Could you check a few things on this model? Use its own coordinates, in mm. A direction names the side the tool comes from. Coordinates: 2 decimals unless noted, no trailing zeros.
from build123d import *

# Parameters (mm, degrees)
F1_DEPTH = 25
F2_D     = 28
F2_DEPTH = 17
F2_TIP   = 8.4120486664
F3_D     = 28
F3_DEPTH = 17
F3_TIP   = 8.4120486664
F4_R     = 10
F5_DEPTH = 25


with BuildPart() as f1:
    # F0 (on Front) → F1 (new body)
    with BuildSketch(Plane.XZ):
        with BuildLine():
            Line((-279.2028378171, 167.9137703829), (54.3474347586, 546.1242293713))
            ThreePointArc((54.3474347586, 546.1242293713), (45.905243427, 563.8289204578), (52.8386613021, 582.1770647105))
            Line((52.8386613021, 582.1770647105), (-362.0687545083, 149.4799000496))
            ThreePointArc((-362.0687545083, 149.4799000496), (-347.0310263397, 160.2264674692), (-329.1166074138, 164.7757063423))
            Line((-329.1166074138, 164.7757063423), (-279.2028378171, 167.9137703829))
        make_face()
        with BuildLine():
            ThreePointArc((70.8833804527, 539.8742293713), (62.0445456879, 541.488870704), (54.3474347586, 546.1242293713))
            Line((54.3474347586, 546.1242293713), (-279.2028378171, 167.9137703829))
            Line((-279.2028378171, 167.9137703829), (-215.3865282422, 171.9258830303))
            Line((-215.3865282422, 171.9258830303), (-35.7808883073, 393.5494389695))
            Line((-35.7808883073, 393.5494389695), (70.8833804527, 525.16732437))
            Line((70.8833804527, 525.16732437), (70.8833804527, 539.8742293713))
        make_face()
        with BuildLine():
            Line((-215.3865282422, 171.9258830303), (-279.2028378171, 167.9137703829))
            Line((-279.2028378171, 167.9137703829), (-292.9074248186, 152.3742293713))
            ThreePointArc((-292.9074248186, 152.3742293713), (-281.7851423828, 138.2595880387), (-276.3714791245, 121.1242293713))
            Line((-276.3714791245, 121.1242293713), (-254.3034374995, 123.904541279))
            Line((-254.3034374995, 123.904541279), (-215.3865282422, 171.9258830303))
        make_face()
        with BuildLine():
            Line((-35.7808883073, 393.5494389695), (-215.3865282422, 171.9258830303))
            Line((-215.3865282422, 171.9258830303), (69.3147348493, 189.8249678568))
            ThreePointArc((69.3147348493, 189.8249678568), (-49.7750455866, 257.3601064033), (-35.7808883073, 393.5494389695))
        make_face()
        with BuildLine():
            Line((54.3474347586, 546.1242293713), (61.788610321, 554.5617293713))
            ThreePointArc((61.788610321, 554.5617293713), (65.226110321, 577.4064995031), (84.6333804527, 564.8742293713))
            ThreePointArc((84.6333804527, 564.8742293713), (80.6060986941, 555.15151113), (70.8833804527, 551.1242293713))
            Line((70.8833804527, 551.1242293713), (70.8833804527, 539.8742293713))
            ThreePointArc((70.8833804527, 539.8742293713), (81.64190304, 542.3075683037), (90.3060950779, 549.1338940322))
            ThreePointArc((90.3060950779, 549.1338940322), (94.4478437994, 556.5246145787), (95.8833804527, 564.8742293713))
            ThreePointArc((95.8833804527, 564.8742293713), (80.2075968068, 588.0703279524), (52.8386613021, 582.1770647105))
            ThreePointArc((52.8386613021, 582.1770647105), (45.905243427, 563.8289204578), (54.3474347586, 546.1242293713))
        make_face()
        with BuildLine():
            ThreePointArc((70.8833804527, 551.1242293713), (66.0220213321, 552.0122821043), (61.788610321, 554.5617293713))
            Line((61.788610321, 554.5617293713), (54.3474347586, 546.1242293713))
            ThreePointArc((54.3474347586, 546.1242293713), (62.0445456879, 541.488870704), (70.8833804527, 539.8742293713))
            Line((70.8833804527, 539.8742293713), (70.8833804527, 551.1242293713))
        make_face()
        with BuildLine():
            Line((70.8833804527, 551.1242293713), (70.8833804527, 564.8742293713))
            Line((70.8833804527, 564.8742293713), (61.788610321, 554.5617293713))
            ThreePointArc((61.788610321, 554.5617293713), (66.0220213321, 552.0122821043), (70.8833804527, 551.1242293713))
        make_face()
        with BuildLine():
            Line((61.788610321, 554.5617293713), (70.8833804527, 564.8742293713))
            Line((70.8833804527, 564.8742293713), (70.8833804527, 551.1242293713))
            ThreePointArc((70.8833804527, 551.1242293713), (80.6060986941, 555.15151113), (84.6333804527, 564.8742293713))
            ThreePointArc((84.6333804527, 564.8742293713), (65.226110321, 577.4064995031), (61.788610321, 554.5617293713))
        make_face()
        with BuildLine():
            Line((69.3147348493, 189.8249678568), (-215.3865282422, 171.9258830303))
            Line((-215.3865282422, 171.9258830303), (-254.3034374995, 123.904541279))
            Line((-254.3034374995, 123.904541279), (46.0794619115, 161.7492293713))
            ThreePointArc((46.0794619115, 161.7492293713), (51.6235827444, 180.8134951083), (69.3147348493, 189.8249678568))
        make_face()
        with BuildLine():
            Line((-325.9793162069, 114.8742293713), (-306.136181374, 137.3742293713))
            ThreePointArc((-306.136181374, 137.3742293713), (-353.3224510399, 102.5310945383), (-295.9793162069, 114.8742293713))
            ThreePointArc((-295.9793162069, 114.8742293713), (-296.0381984298, 116.7529167476), (-296.2146139575, 118.6242293713))
            Line((-296.2146139575, 118.6242293713), (-325.9793162069, 114.8742293713))
        make_face()
        with BuildLine():
            Line((-306.136181374, 137.3742293713), (-292.9074248186, 152.3742293713))
            ThreePointArc((-292.9074248186, 152.3742293713), (-309.7784140786, 162.1767744427), (-329.1166074138, 164.7757063423))
            ThreePointArc((-329.1166074138, 164.7757063423), (-347.0310263397, 160.2264674692), (-362.0687545083, 149.4799000496))
            ThreePointArc((-362.0687545083, 149.4799000496), (-369.9271571596, 91.0291612104), (-316.6410453648, 65.7540024004))
            ThreePointArc((-316.6410453648, 65.7540024004), (-300.3237958419, 71.9580986651), (-287.1338869566, 83.3935586931))
            ThreePointArc((-287.1338869566, 83.3935586931), (-278.8503895137, 98.1749997861), (-275.9793162069, 114.8742293713))
            ThreePointArc((-275.9793162069, 114.8742293713), (-276.0774532451, 118.0053749985), (-276.3714791245, 121.1242293713))
            Line((-276.3714791245, 121.1242293713), (-296.2146139575, 118.6242293713))
            ThreePointArc((-296.2146139575, 118.6242293713), (-296.0381984298, 116.7529167476), (-295.9793162069, 114.8742293713))
            ThreePointArc((-295.9793162069, 114.8742293713), (-353.3224510399, 102.5310945383), (-306.136181374, 137.3742293713))
        make_face()
        with BuildLine():
            ThreePointArc((-276.3714791245, 121.1242293713), (-281.7851423828, 138.2595880387), (-292.9074248186, 152.3742293713))
            Line((-292.9074248186, 152.3742293713), (-306.136181374, 137.3742293713))
            ThreePointArc((-306.136181374, 137.3742293713), (-299.4628119124, 128.9054445717), (-296.2146139575, 118.6242293713))
            Line((-296.2146139575, 118.6242293713), (-276.3714791245, 121.1242293713))
        make_face()
        with BuildLine():
            Line((-292.9074248186, 152.3742293713), (-279.2028378171, 167.9137703829))
            Line((-279.2028378171, 167.9137703829), (-329.1166074138, 164.7757063423))
            ThreePointArc((-329.1166074138, 164.7757063423), (-309.7784140786, 162.1767744427), (-292.9074248186, 152.3742293713))
        make_face()
        with BuildLine():
            Line((-254.3034374995, 123.904541279), (-276.3714791245, 121.1242293713))
            ThreePointArc((-276.3714791245, 121.1242293713), (-276.0774532451, 118.0053749985), (-275.9793162069, 114.8742293713))
            ThreePointArc((-275.9793162069, 114.8742293713), (-278.8503895137, 98.1749997861), (-287.1338869566, 83.3935586931))
            Line((-287.1338869566, 83.3935586931), (-254.3034374995, 123.904541279))
        make_face()
        with BuildLine():
            Line((46.0794619115, 161.7492293713), (-254.3034374995, 123.904541279))
            Line((-254.3034374995, 123.904541279), (-287.1338869566, 83.3935586931))
            ThreePointArc((-287.1338869566, 83.3935586931), (-300.3237958419, 71.9580986651), (-316.6410453648, 65.7540024004))
            Line((-316.6410453648, 65.7540024004), (75.5525158738, 140.3141158858))
            ThreePointArc((75.5525158738, 140.3141158858), (56.1790139122, 144.6558811539), (46.0794619115, 161.7492293713))
        make_face()
        with BuildLine():
            ThreePointArc((-296.2146139575, 118.6242293713), (-299.4628119124, 128.9054445717), (-306.136181374, 137.3742293713))
            Line((-306.136181374, 137.3742293713), (-325.9793162069, 114.8742293713))
            Line((-325.9793162069, 114.8742293713), (-296.2146139575, 118.6242293713))
        make_face()
        with BuildLine():
            ThreePointArc((70.8833804527, 189.8742293713), (70.098670996, 189.8619109578), (69.3147348493, 189.8249678568))
            ThreePointArc((69.3147348493, 189.8249678568), (51.6235827444, 180.8134951083), (46.0794619115, 161.7492293713))
            Line((46.0794619115, 161.7492293713), (57.2412252551, 163.1554793713))
            ThreePointArc((57.2412252551, 163.1554793713), (60.5708804527, 173.9689995031), (70.8833804527, 178.6242293713))
            Line((70.8833804527, 178.6242293713), (70.8833804527, 189.8742293713))
        make_face()
        with BuildLine():
            ThreePointArc((70.8833804527, 178.6242293713), (60.5708804527, 173.9689995031), (57.2412252551, 163.1554793713))
            Line((57.2412252551, 163.1554793713), (70.8833804527, 164.8742293713))
            Line((70.8833804527, 164.8742293713), (70.8833804527, 178.6242293713))
        make_face()
        with BuildLine():
            Line((70.8833804527, 164.8742293713), (57.2412252551, 163.1554793713))
            ThreePointArc((57.2412252551, 163.1554793713), (71.7444455002, 151.1512170568), (84.6333804527, 164.8742293713))
            ThreePointArc((84.6333804527, 164.8742293713), (80.6060986941, 174.5969476126), (70.8833804527, 178.6242293713))
            Line((70.8833804527, 178.6242293713), (70.8833804527, 164.8742293713))
        make_face()
        with BuildLine():
            Line((57.2412252551, 163.1554793713), (46.0794619115, 161.7492293713))
            ThreePointArc((46.0794619115, 161.7492293713), (56.1790139122, 144.6558811539), (75.5525158738, 140.3141158858))
            ThreePointArc((75.5525158738, 140.3141158858), (90.1412150341, 148.9325918382), (95.8833804527, 164.8742293713))
            ThreePointArc((95.8833804527, 164.8742293713), (88.5610499824, 182.551898901), (70.8833804527, 189.8742293713))
            Line((70.8833804527, 189.8742293713), (70.8833804527, 178.6242293713))
            ThreePointArc((70.8833804527, 178.6242293713), (80.6060986941, 174.5969476126), (84.6333804527, 164.8742293713))
            ThreePointArc((84.6333804527, 164.8742293713), (71.7444455002, 151.1512170568), (57.2412252551, 163.1554793713))
        make_face()
        with BuildLine():
            ThreePointArc((90.3060950779, 549.1338940322), (81.64190304, 542.3075683037), (70.8833804527, 539.8742293713))
            Line((70.8833804527, 539.8742293713), (70.8833804527, 525.16732437))
            Line((70.8833804527, 525.16732437), (90.3060950779, 549.1338940322))
        make_face()
    extrude(amount=F1_DEPTH)

    # F2
    with Locations(Plane(origin=(0, 0, 0), x_dir=(1, 0, 0), z_dir=(0, 1, 0))):
        with Locations((70.8833804527, -564.8742293713)):
            Hole(F2_D / 2, depth=F2_DEPTH)
            with Locations((0, 0, -(F2_DEPTH + F2_TIP / 2))):  # 118° drill point
                Cone(0, F2_D / 2, F2_TIP, mode=Mode.SUBTRACT)

    # F3
    with Locations(Plane(origin=(0, 0, 0), x_dir=(1, 0, 0), z_dir=(0, 1, 0))):
        with Locations((70.8833804527, -164.8742293713)):
            Hole(F3_D / 2, depth=F3_DEPTH)
            with Locations((0, 0, -(F3_DEPTH + F3_TIP / 2))):  # 118° drill point
                Cone(0, F3_D / 2, F3_TIP, mode=Mode.SUBTRACT)

    # F4
    f4_edges = [f1.edges().sort_by_distance(p)[0] for p in [
        (-49.775046, 0, 257.360106),
        (95.687299, 0, 167.999229),
    ]]
    fillet(f4_edges, radius=F4_R)

    # F0 (on Front) → F5 (join)
    with BuildSketch(Plane.XZ):
        with BuildLine():
            Line((-325.9793162069, 114.8742293713), (-306.136181374, 137.3742293713))
            ThreePointArc((-306.136181374, 137.3742293713), (-353.3224510399, 102.5310945383), (-295.9793162069, 114.8742293713))
            ThreePointArc((-295.9793162069, 114.8742293713), (-296.0381984298, 116.7529167476), (-296.2146139575, 118.6242293713))
            Line((-296.2146139575, 118.6242293713), (-325.9793162069, 114.8742293713))
        make_face()
        with BuildLine():
            ThreePointArc((-296.2146139575, 118.6242293713), (-299.4628119124, 128.9054445717), (-306.136181374, 137.3742293713))
            Line((-306.136181374, 137.3742293713), (-325.9793162069, 114.8742293713))
            Line((-325.9793162069, 114.8742293713), (-296.2146139575, 118.6242293713))
        make_face()
    extrude(amount=F5_DEPTH)


solid = f1.part
1) Will these pins go through, and if not, where does the flat tip stop? pin 1 (3 mm diameter, centred on x = -328.5, y = -19.5, fed in from +Z); pin 2 (10 mm diameter, centred on y = -13.5, z = 398.5, fed in from -X); pin 3 (1.5 mm diameter, centred on y = -14, z = 146, fed in from +X).
2) We'd pull the mould along X, two halves only. Please class faces 5 (the flat face through (-123.29, -17.395, 102.512)), 6 (the flat face through (-124, -25, 251)), 7 (the conical face through (69.76, -24.5, 163.85)): released by +X, released by -X, zero draft, split by the parting line, or undercut.
3) If I drill on L1, parallel to Z at x = 29, y = -23.25; L2, parallel to Z at x = -11.5, y = -7.75; L3, parallel to Z at x = -80, y = -12.25, over which ranges is the centre line in solid material (lowest first)?
4) For faces 1 (the cylindrical face through (-118.331, -3.007, 106.357)), 2 (the cylindrical face through (25.9, -3, 474.2)), 3 (the cylindrical face through (63.357, -8.619, 153.069)), 4 (the flat face through (26.38, -17.4, 470.25)), which set-ups out of +Z, -Z, +X, -X, +Y, -Y let a thin tool reach every point of the face, with its end or its side?
Solved:
1. pin 1: stops at z = 186.05
1. pin 2: stops at x = -128.08
1. pin 3: stops at x = 88.1
2. face 5: released by +X
2. face 6: zero draft
2. face 7: undercut
3. L1: z = 131.46 to 193.86, 473.49 to 557.32
3. L2: z = 124.03 to 212.73, 423.92 to 514.71
3. L3: z = 110.74 to 443.64
4. face 1: -Z, +X, +Y
4. face 2: +X, +Y
4. face 3: +Y
4. face 4: +X, +Y, -Y
